```python
from build123d import *

# Parameters (mm, degrees)
SKETCH_1_R                           = 2.25
EXTRUDE_1_DEPTH                      = 80
EXTRUDE_3_DEPTH                      = 0.75
CHAMFER_4_SIZE                       = 0.7
PATTERN_CIRCULAR_1_COUNT             = 6
CHAMFER_4_OF_PATTERN_CIRCULAR_1_SIZE = 0.7
SKETCH_7_R                           = 3
EXTRUDE_4_DEPTH                      = 8
CHAMFER_6_SIZE                       = 1
CHAMFER_7_SIZE                       = 0.7
SKETCH_8_R                           = 1.5
CUT_EXTRUDE_3_DEPTH                  = 75
SKETCH_9_R                           = 2
CUT_EXTRUDE_4_DEPTH                  = 1
CHAMFER_8_SIZE                       = 1


# Some blends are built 0.0001 mm under size
with BuildPart() as part:
    # 스케치1 → 보스-돌출1 (new body)
    with BuildSketch(Plane.XY):
        Circle(SKETCH_1_R)
    extrude(amount=EXTRUDE_1_DEPTH)

    # 스케치5 → 보스-돌출3 (add, symmetric)
    with BuildSketch(Plane(origin=(0, 0, 0), x_dir=(0, 0, -1), z_dir=(1, 0, 0))):
        Polygon((0, 1.323110618), (0, 5.8), (-12.84952222, 5.8), (-30, 1.323110618), align=None)
    extrude_3 = extrude(amount=EXTRUDE_3_DEPTH, both=True)

    # 모따기4
    chamfer_4_edges = [part.edges().sort_by_distance(p)[0] for p in [
        (-0.75, 3.960660172, 19.895833657),
        (-0.75, 5.8, 6.42476111),
        (0.75, 5.8, 6.42476111),
        (0.75, 3.960660172, 19.895833657),
    ]]
    chamfer(chamfer_4_edges, length=CHAMFER_4_SIZE)

    # 원형 패턴1: 보스-돌출3 ×6 about axis
    pattern_circular_1_axis = Axis((0, 0, 0), (0, 0, 1))
    for i in range(1, PATTERN_CIRCULAR_1_COUNT):
        add(extrude_3.rotate(pattern_circular_1_axis, i * 360 / PATTERN_CIRCULAR_1_COUNT))

    # 모따기4 of 원형 패턴1
    chamfer_4_of_pattern_circular_1_edges = [part.edges().sort_by_distance(p)[0] for p in [
        (-3.805032325, 1.330811033, 19.895833657),
        (-5.397947342, 2.250480947, 6.42476111),
        (-4.647947342, 3.549519053, 6.42476111),
        (-3.055032325, 2.629849139, 19.895833657),
        (-3.055032325, -2.629849139, 19.895833657),
        (-4.647947342, -3.549519053, 6.42476111),
        (-5.397947342, -2.250480947, 6.42476111),
        (-3.805032325, -1.330811033, 19.895833657),
        (0.75, -3.960660172, 19.895833657),
        (0.75, -5.8, 6.42476111),
        (-0.75, -5.8, 6.42476111),
        (-0.75, -3.960660172, 19.895833657),
        (3.805032325, -1.330811033, 19.895833657),
        (5.397947342, -2.250480947, 6.42476111),
        (4.647947342, -3.549519053, 6.42476111),
        (3.055032325, -2.629849139, 19.895833657),
        (3.055032325, 2.629849139, 19.895833657),
        (4.647947342, 3.549519053, 6.42476111),
        (5.397947342, 2.250480947, 6.42476111),
        (3.805032325, 1.330811033, 19.895833657),
    ]]
    chamfer(chamfer_4_of_pattern_circular_1_edges, length=CHAMFER_4_OF_PATTERN_CIRCULAR_1_SIZE)

    # 스케치7 → 보스-돌출4 (add)
    with BuildSketch(Plane.XY.offset(80)):
        Circle(SKETCH_7_R)
    extrude(amount=EXTRUDE_4_DEPTH)

    # 모따기6
    # the kernel refuses this chamfer: 1 mm, written as the material it adds along each edge
    with BuildSketch(Plane(origin=(0, 0, 80), x_dir=(1, 0, 0), z_dir=(0, -1, 0))) as chamfer_6_piece_1_section:
        Polygon((2.25 + CHAMFER_6_SIZE, 0), (2.25, -CHAMFER_6_SIZE), (2.25, 0), align=None)
    chamfer_6_piece_1 = revolve(axis=Axis((0, 0, 80), (0, 0, 1)), mode=Mode.PRIVATE)
    chamfer_6_piece_1 = chamfer_6_piece_1 & Plane(origin=(0, 0, 79.375065252), x_dir=(1, 0, 0), z_dir=(0, 0, -1)) * Cylinder(3, 13, mode=Mode.PRIVATE)
    add(chamfer_6_piece_1)

    # 모따기7
    chamfer_7_edges = [part.edges().sort_by_distance(p)[0] for p in [
        (-3, 0, 88),
    ]]
    chamfer(chamfer_7_edges, length=CHAMFER_7_SIZE)

    # 스케치8 → 컷-돌출3 (cut)
    with BuildSketch(Plane.XY.offset(88)):
        Circle(SKETCH_8_R)
    extrude(amount=-CUT_EXTRUDE_3_DEPTH, mode=Mode.SUBTRACT)

    # 스케치9 → 컷-돌출4 (cut)
    with BuildSketch(Plane.XY):
        Circle(SKETCH_9_R)
    extrude(amount=CUT_EXTRUDE_4_DEPTH, mode=Mode.SUBTRACT)

    # 모따기8
    chamfer_8_edges = [part.edges().sort_by_distance(p)[0] for p in [
        (-2, 0, 1),
    ]]
    chamfer(chamfer_8_edges, length=CHAMFER_8_SIZE - 0.0001)  # a hair under: the kernel refuses the full size


solid = part.part
```
Here's how the part is built. I have some questions about the finished solid (model axes, mm). A direction names the side the tool comes from. Give positions to 0.01 mm unless a question says otherwise; leave off trailing zeros. Write each loop counter-clockwise with the first axis right and the second up, starting at its lowest first coordinate (ties: lowest second). Pieces come first, ordered by that corner, then holes.
(1) Imagine slicing it at A-A, the plane z = 73.5. Write out the boundary of the cut face in (x, y), and give its area (3 significant figures).
Output values:
outline: circle Ø4.5 at (0, 0); hole circle Ø3 at (0, 0)
area: 8.84 mm2
(2) Thinking about a two-plate mould opening in Y: for faces 4 (the face through (3.415, -1.516, 19.468)), 5 (the face through (2.77, 2.465, 9.569)), 6 (the face through (0.75, -4, 10)), 7 (the face through (-0.4, -3.7, 19.5)), which applies, pulls with the +Y half, pulls with the -Y half, needs draft (parallel to the pull), parting line crosses it, or undercut?
Output values:
face 4: undercut
face 5: pulls with the +Y half
face 6: needs draft
face 7: pulls with the -Y half
(3) If I drill on L1, parallel to Y at x = 0, z = 66; L2, parallel to X at y = 0, z = 0.05; L3, parallel to X at y = 3.5, z = 18, over which ranges is the centre line in solid material (lowest first)?
Output values:
L1: y = -2.25 to -1.5, 1.5 to 2.25
L2: x = -2.25 to -1.95, 1.95 to 2.25
L3: x = -0.75 to 0.75
(4) On a 3-axis mill with a long thin cutter (end or side, diameter ignored), from which of +Z, -Z, +X, -X, +Y, -Y can I reach the whole of each face in a straight line? I mean faces 1 (the face through (0, 0, 1)), 2 (the face through (0, 0, 13)), 3 (the face through (-3.415, 1.516, 19.468)). Say none if no direction works.
Output values:
face 1: -Z
face 2: +Z
face 3: -X
(5) Will these pins go through, and if not, where does the flat tip stop? pin 1 (1.5 mm diameter, centred on y = -4, z = 13, fed in from -X); pin 2 (0.9 mm diameter, centred on x = 0, y = -0.5, fed in from +Z); pin 3 (2 mm diameter, centred on x = 0.5, y = 0, fed in from -Z).
Output values:
pin 1: stops at x = -0.75
pin 2: stops at z = 13
pin 3: stops at z = 0.5
